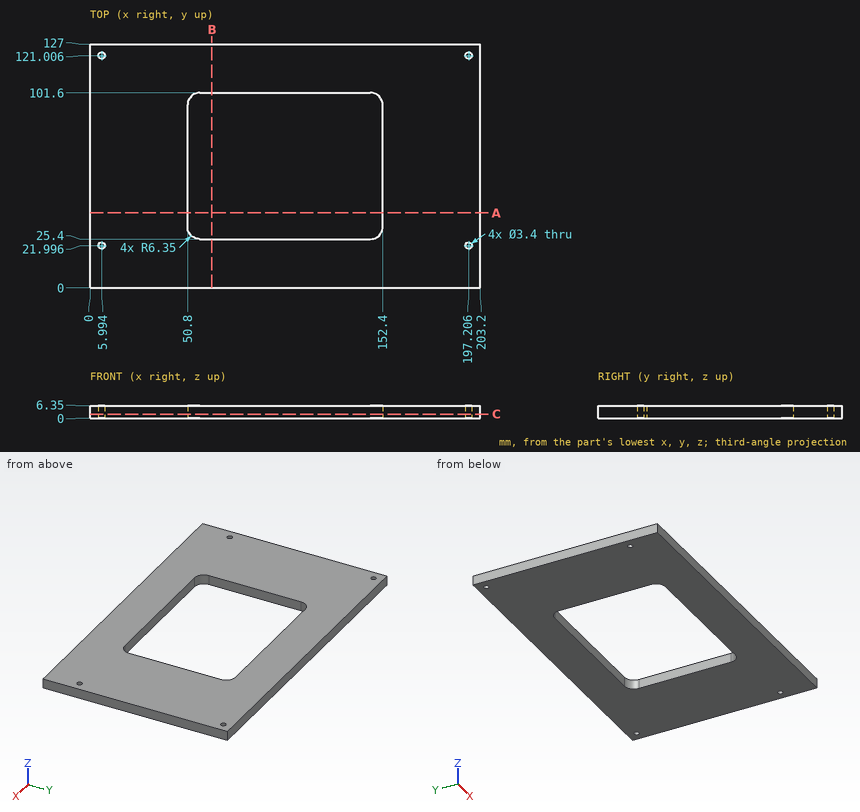
Geometry check sheet. Reference: drawing and pictorial views, mm from the part's lowest x, y, z. Give positions to 0.01 mm unless a question says otherwise; leave off trailing zeros. Loops run counter-clockwise (first coordinate to the right, second up) from the corner with the lowest first, then second, coordinate; pieces in that order, holes last.
1. Section check C-C, the plane z = 2. Count the separate pieces of the cut face and the enclosed holes in it, then the cut area to 3 significant figures.
2. Thickness scan on line 1 (X direction, y = 91, z = 5); line 2 (Y direction, x = 136, z = 5.25); line 3 (X direction, y = 96.5, z = 3.25) (1 decimal). Record the ranges inside material, lowest first.
3. Section check A-A, the plane y = 39. Enter the section's corners in (x, z).
4. Section check B-B, the plane x = 63.5. Enter the section's corners in (y, z).
Geometry says:
1. separate pieces: 1
1. enclosed holes: 5
1. area: 18,100 mm2
2. line 1: x = 0 to 50.8, 152.4 to 203.2
2. line 2: y = 0 to 25.4, 101.6 to 127
2. line 3: x = 0 to 50.9, 152.3 to 203.2
3. outline: (0, 0) - (50.8, 0) - (50.8, 6.35) - (0, 6.35) - close; (152.4, 0) - (203.2, 0) - (203.2, 6.35) - (152.4, 6.35) - close
4. outline: (0, 0) - (25.4, 0) - (25.4, 6.35) - (0, 6.35) - close; (101.6, 0) - (127, 0) - (127, 6.35) - (101.6, 6.35) - close
